Model file for the job. Use its own axes, mm. A direction names the side the tool comes from. Coordinates: 2 decimals unless noted, no trailing zeros. Loops run counter-clockwise (first coordinate to the right, second up) from the corner with the lowest first, then second, coordinate; pieces in that order, holes last.
from build123d import *

# Parameters (mm, degrees)
PAD_DEPTH         = 12
PAD001_DEPTH      = 12
SKETCH001_R       = 3
POCKET_DEPTH      = 255.365913
POCKET_DEPTH_BACK = 207.701119
FILLET_R          = 7.9


with BuildPart() as part:
    # Sketch → Pad (new body)
    with BuildSketch(Plane.XY):
        with BuildLine():
            ThreePointArc((0, 28), (-19.79899, 19.79899), (-28, 0))
            Line((-32.664794, 0), (-28, 0))
            ThreePointArc((-32.664794, 0), (-38.664794, 6), (-44.664794, 0))
            Line((-47.664794, 0), (-44.664794, 0))
            Line((-47.664794, 9), (-47.664794, 0))
            Line((-29.664794, 9), (-47.664794, 9))
            ThreePointArc((-4, 30.740852), (-20.037359, 23.653842), (-29.664794, 9))
            Line((-4, 30.740852), (-4, 45.740852))
            Line((-4, 45.740852), (0, 45.740852))
            Line((0, 45.740852), (0, 28))
        make_face()
    extrude(amount=PAD_DEPTH)

    # Sketch → Pad001 (join)
    with BuildSketch(Plane.XY):
        with BuildLine():
            ThreePointArc((0, 28), (-19.79899, 19.79899), (-28, 0))
            Line((-32.664794, 0), (-28, 0))
            ThreePointArc((-32.664794, 0), (-38.664794, 6), (-44.664794, 0))
            Line((-47.664794, 0), (-44.664794, 0))
            Line((-47.664794, 9), (-47.664794, 0))
            Line((-29.664794, 9), (-47.664794, 9))
            ThreePointArc((-4, 30.740852), (-20.037359, 23.653842), (-29.664794, 9))
            Line((-4, 30.740852), (-4, 45.740852))
            Line((-4, 45.740852), (0, 45.740852))
            Line((0, 45.740852), (0, 28))
        make_face()
    pad001 = extrude(amount=PAD001_DEPTH)

    # Mirrored001: Pad001 across Sketch H_Axis
    add(pad001.mirror(Plane.ZX))

    # Sketch001 → Pocket (cut, two sides)
    with BuildSketch(Plane.YZ) as pocket_sk:
        with Locations((-38, 6)):
            Circle(SKETCH001_R)
    pocket = extrude(amount=-POCKET_DEPTH, mode=Mode.SUBTRACT) + extrude(pocket_sk.sketch, amount=POCKET_DEPTH_BACK, mode=Mode.SUBTRACT)

    # Mirrored: Pocket across Sketch001 V_Axis
    add(pocket.mirror(Plane(origin=(0, 0, 0), x_dir=(1, 0, 0), z_dir=(0, 1, 0))), mode=Mode.SUBTRACT)

    # Fillet
    fillet_edges = [part.edges().sort_by_distance(p)[0] for p in [
        (-47.664794, 9, 6),
        (-47.664794, -9, 6),
        (-29.664794, -9, 6),
        (-29.664794, 9, 6),
    ]]
    fillet(fillet_edges, radius=FILLET_R)


solid = part.part
Q1. Mould opens along Y. For faces 1 (the cylindrical face through (-17.97, -25.26, 5.92)), 2 (the flat face through (0, -35, 5)), 3 (the cylindrical face through (-2, -41, 6)) say: +Y half, -Y half, draft (parallel to the pull), parting line (faces both ways), or undercut.
Answers:
face 1: -Y half
face 2: draft
face 3: undercut
Q2. Flat gauge pins, fed straight in: P1, Ø7, axis at x = -38.66, y = 0, coming from the +Z side; P2, Ø3, axis at x = -39.5, z = 5, coming from the -Y side; P3, Ø6, axis at y = -36, z = 4, coming from the -X side; P4, Ø1, axis at y = -26, z = 2, coming from the -X side. Where does each tip first touch, or does it go through?
Answers:
P1: passes through
P2: stops at y = -9
P3: stops at x = -4
P4: stops at x = -17.63
Q3. Slice it at B-B (z = 6). List the corners of the cut face in (x, y).
Answers:
outline: (-47.66, -1.1) arc R7.9 ccw to (-39.76, -9) - (-35.04, -9) arc R7.9 cw to (-27.92, -13.47) arc R31 ccw to (-4, -30.74) - (-4, -35) - (0, -35) - (0, -28) arc R28 cw to (0, 28) - (0, 35) - (-4, 35) - (-4, 30.74) arc R31 ccw to (-27.92, 13.47) arc R7.9 cw to (-35.04, 9) - (-39.76, 9) arc R7.9 ccw to (-47.66, 1.1) - close; (-4, -45.74) - (0, -45.74) - (0, -41) - (-4, -41) - close; (-4, 41) - (0, 41) - (0, 45.74) - (-4, 45.74) - close; hole circle Ø12 at (-38.66, 0)
Q4. Slice it at C-C (x = -15.5). List the corners of the cut face in (y, z), and give its area (3 significant figures).
Answers:
outline: (-26.85, 0) - (-23.32, 0) - (-23.32, 12) - (-26.85, 12) - close; (23.32, 0) - (26.85, 0) - (26.85, 12) - (23.32, 12) - close
area: 84.7 mm2
Q5. Slice it at A-A (y = -38). List the corners of the cut face in (x, z).
Answers:
outline: (-4, 0) - (0, 0) - (0, 3) - (-4, 3) - close; (-4, 9) - (0, 9) - (0, 12) - (-4, 12) - close
Q6. Drill centre lines: line 1 (X direction, y = 0, z = 8.5); line 2 (Z direction, x = -1, y = 38); line 3 (X direction, y = 31.5, z = 8.25). Where is each one in solid material? Low to high.
Answers:
line 1: x = -47.66 to -44.66, -32.66 to -28
line 2: z = 0 to 3, 9 to 12
line 3: x = -4 to 0
Q7. Which spindle directions (+Z, -Z, +X, -X, +Y, -Y) get a long thin tool onto all of the face, cutting with end or side? Do faces 4 (the cylindrical face through (-33.122, -2.298, 5.916)), 5 (the flat face through (-37, -9, 6)), 6 (the flat face through (-37, 9, 6)). Say none if no direction does.
Answers:
face 4: +Z, -Z
face 5: +Z, -Z, -X, -Y
face 6: +Z, -Z, -X, +Y
Q8. Slice it at D-D (z = 10.25). List the corners of the cut face in (x, y), and give its area (3 significant figures).
Answers:
outline: (-47.66, -1.1) arc R7.9 ccw to (-39.76, -9) - (-35.04, -9) arc R7.9 cw to (-27.92, -13.47) arc R31 ccw to (-4, -30.74) - (-4, -45.74) - (0, -45.74) - (0, -28) arc R28 cw to (0, 28) - (0, 45.74) - (-4, 45.74) - (-4, 30.74) arc R31 ccw to (-27.92, 13.47) arc R7.9 cw to (-35.04, 9) - (-39.76, 9) arc R7.9 ccw to (-47.66, 1.1) - close; hole circle Ø12 at (-38.66, 0)
area: 574 mm2
